Work out the finished part from the listing and answer in its coordinate system (mm). A direction names the side the tool comes from. Round coordinates to 2 decimals unless told otherwise and drop trailing zeros. Loops run counter-clockwise (first coordinate to the right, second up) from the corner with the lowest first, then second, coordinate; pieces in that order, holes last. Notation, with made-up numbers: (-10, 25.5) -> (49, 25.5) arc R21 ccw to (49, 41.5) -> close; hole circle Ø11 at (42.25, -5). An arc over 180 degrees is marked (long way). Use one line per item in the form item = value.
```python
from build123d import *

# Parameters (mm, degrees)
BOSS_EXTRUDE1_DEPTH = 100
FILLET1_R           = 1
BOSS_EXTRUDE2_START = 2.5
BOSS_EXTRUDE2_DEPTH = 2.5


with BuildPart() as part:
    # Sketch1 → Boss-Extrude1 (new body)
    with BuildSketch(Plane(origin=(0, 0, 0), x_dir=(1, 0, 0), z_dir=(0, 1, 0))):
        with BuildLine():
            Line((-147.5, 118.765325103), (-145, 118.765325103))
            Line((-145, 118.765325103), (-145, 81.265325103))
            Line((-145, 81.265325103), (-125, 81.265325103))
            Line((-125, 81.265325103), (125, 81.265325103))
            Line((125, 81.265325103), (145, 81.265325103))
            Line((145, 81.265325103), (145, 118.765325103))
            Line((145, 118.765325103), (147.5, 118.765325103))
            Line((147.5, 118.765325103), (147.5, 78.765325103))
            Line((147.5, 78.765325103), (127.5, 78.765325103))
            Line((127.5, 78.765325103), (127.5, -101.234674897))
            Line((127.5, -101.234674897), (147.5, -101.234674897))
            Line((147.5, -101.234674897), (147.5, -150.264700033))
            ThreePointArc((147.5, -150.264700033), (0, -210.560514048), (-147.5, -150.264700033))
            Line((-147.5, -150.264700033), (-147.5, -101.234674897))
            Line((-147.5, -101.234674897), (-127.5, -101.234674897))
            Line((-127.5, -101.234674897), (-127.5, 78.765325103))
            Line((-127.5, 78.765325103), (-147.5, 78.765325103))
            Line((-147.5, 78.765325103), (-147.5, 118.765325103))
        make_face()
        with BuildLine():
            Line((145, -149.211854441), (145, -103.734674897))
            Line((145, -103.734674897), (125, -103.734674897))
            Line((125, -103.734674897), (125, 78.765325103))
            Line((125, 78.765325103), (-125, 78.765325103))
            Line((-125, 78.765325103), (-125, -103.734674897))
            Line((-125, -103.734674897), (-145, -103.734674897))
            Line((-145, -103.734674897), (-145, -149.211854441))
            ThreePointArc((-145, -149.211854441), (0, -208.060514048), (145, -149.211854441))
        make_face(mode=Mode.SUBTRACT)
    extrude(amount=BOSS_EXTRUDE1_DEPTH)

    # Fillet1
    fillet1_edges = [part.edges().sort_by_distance(p)[0] for p in [
        (-146.25, 0, -118.765325103),
        (146.25, 100, -118.765325103),
        (146.25, 0, -118.765325103),
        (147.5, 50, 101.234674897),
        (-147.5, 50, 150.264700033),
        (-127.5, 50, 101.234674897),
        (-127.5, 50, -78.765325103),
        (-147.5, 50, -78.765325103),
        (145, 50, -81.265325103),
        (145, 50, -118.765325103),
        (147.5, 50, -118.765325103),
        (147.5, 50, -78.765325103),
        (127.5, 50, 101.234674897),
        (-146.25, 100, -118.765325103),
        (-145, 50, 103.734674897),
        (145, 50, 149.211854441),
    ]]
    fillet(fillet1_edges, radius=FILLET1_R)

    # Sketch4 → Boss-Extrude2 (add)
    with BuildSketch(Plane(origin=(0, 0, 0), x_dir=(1, 0, 0), z_dir=(0, 1, 0)).offset(BOSS_EXTRUDE2_START)):
        with BuildLine():
            Line((147.5, 79.765325103), (147.5, 117.765325103))
            Line((147.5, 117.765325103), (145, 117.765325103))
            Line((145, 117.765325103), (145, 82.265325103))
            ThreePointArc((145, 82.265325103), (144.707106781, 81.558218322), (144, 81.265325103))
            Line((144, 81.265325103), (-145, 81.265325103))
            Line((-145, 81.265325103), (-145, 117.765325103))
            Line((-145, 117.765325103), (-147.5, 117.765325103))
            Line((-147.5, 117.765325103), (-147.5, 79.765325103))
            ThreePointArc((-147.5, 79.765325103), (-147.207106781, 79.058218322), (-146.5, 78.765325103))
            Line((-146.5, 78.765325103), (-128.5, 78.765325103))
            ThreePointArc((-128.5, 78.765325103), (-127.792893219, 78.472431884), (-127.5, 77.765325103))
            Line((-127.5, 77.765325103), (-127.5, -100.234674897))
            ThreePointArc((-127.5, -100.234674897), (-127.792893219, -100.941781678), (-128.5, -101.234674897))
            Line((-128.5, -101.234674897), (-147.5, -101.234674897))
            Line((-147.5, -101.234674897), (-147.5, -149.844449507))
            ThreePointArc((-147.5, -149.844449507), (-147.421705506, -150.232339904), (-147.19908208, -150.559490936))
            ThreePointArc((-147.19908208, -150.559490936), (0.210626014, -210.560408702), (147.5, -150.264700033))
            Line((147.5, -150.264700033), (147.5, -102.234674897))
            ThreePointArc((147.5, -102.234674897), (147.207106781, -101.527568116), (146.5, -101.234674897))
            Line((146.5, -101.234674897), (128.5, -101.234674897))
            ThreePointArc((128.5, -101.234674897), (127.792893219, -100.941781678), (127.5, -100.234674897))
            Line((127.5, -100.234674897), (127.5, 78.765325103))
            Line((127.5, 78.765325103), (146.5, 78.765325103))
            ThreePointArc((146.5, 78.765325103), (147.207106781, 79.058218322), (147.5, 79.765325103))
        make_face()
    extrude(amount=-BOSS_EXTRUDE2_DEPTH)


solid = part.part
```
(1) For a pull along Z with two mould halves and no side action, classify faces 5 (the cylindrical face through (-2.455, 50.568, 208.046)), 6 (the flat face through (-3, 49, -81.265)), 7 (the flat face through (145, 49, -100)) as +Z half, -Z half, draft (parallel to the pull), parting line (faces both ways), or undercut.
Completed:
face_5 = undercut
face_6 = -Z half
face_7 = draft
(2) Consider L1, parallel to X at y = 6, z = 43.5; L2, parallel to Z at x = 4.5, y = 23.5; L3, parallel to X at y = 16, z = 143.5. Determine where each line is inside the solid, lowest interval first.
Completed:
L1 = -127.5 to -125, 125 to 127.5
L2 = -81.27 to -78.77, 208.01 to 210.51
L3 = -147.5 to -145, 145 to 147.5
(3) For faces 1 (the flat face through (125, 51, 14)), 2 (the flat face through (-145, 49, -100)), 3 (the flat face through (-137, 49, -78.765)), 4 (the flat face through (127.5, 49, 9)), determine the directions among +Z, -Z, +X, -X, +Y, -Y from which every point of the face is accessible in a straight line to the end or side of a thin tool.
Completed:
face_1 = +Y
face_2 = -Z, +Y, -Y
face_3 = -X, +Y, -Y
face_4 = +X, +Y, -Y
(4) Find section A-A, the plane z = 125. Write down the section's boundary in (x, y), then the cut area to 4 significant figures.
Completed:
outline = (-147.5, 0) -> (147.5, 0) -> (147.5, 100) -> (145, 100) -> (145, 2.5) -> (-145, 2.5) -> (-145, 100) -> (-147.5, 100) -> close
area = 1,225 mm2
(5) Given P1, Ø14.5, axis at x = -137.5, y = 59, coming from the +Z side; P2, Ø10, axis at y = 33, z = 52.5, coming from the +X side; P3, Ø9, axis at x = 135, y = 32.5, coming from the -Z side; P4, Ø8, axis at x = -99.5, z = -62, coming from the -Y side, each flat-ended and moving along its own axis, determine where each tip first touches the part or whether it passes through.
Completed:
P1 = 165.44
P2 = 127.5
P3 = -81.27
P4 = 0
(6) Find section B-B, the plane x = 68.5. Write down the section's boundary in (y, z), then the cut area to 3 significant figures.
Completed:
outline = (0, -81.27) -> (100, -81.27) -> (100, -78.77) -> (2.5, -78.77) -> (2.5, 196.46) -> (100, 196.46) -> (100, 199.11) -> (0, 199.11) -> close
area = 1,200 mm2
